Job drawing, mm, ordinate dimensions from the low corner. One solid piece. A direction names the side the tool comes from. Coordinates: 2 decimals unless noted, no trailing zeros. Loops run counter-clockwise (first coordinate to the right, second up) from the corner with the lowest first, then second, coordinate; pieces in that order, holes last. Notation, with made-up numbers: M 61,58 L 117,58 A6 ccw 117,66 Z; hole C -40,47.5 d7. An arc over 180 degrees is marked long. Answer as a JSON object with one key per item and string values. Group by question number.
1. Drill centre lines: L1, parallel to Z at x = 2.5, y = 9; L2, parallel to Z at x = 18.5, y = 13.5; L3, parallel to X at y = 8.95, z = 1.65 (1 decimal). Where is each one in solid material? Low to high.
2. Drop flat-ended pins along their axis: pin 1 Ø8 at (x, z) = (8, 4.5) entering from -Y; pin 2 Ø10 at (x, z) = (23, 3) entering from -Y; pin 3 Ø2 at (x, y) = (7.5, 17) entering from +Z. Give the stop position or say it passes through.
3. 3-axis set-ups, long thin cutter, end or side, ignore diameter. For the marked faces 5, 6 and 7: which of +Z, -Z, +X, -X, +Y, -Y reach the whole face in a straight line?
4. Mould opens along X. For the marked faces 1, 2, 3 and 4 say: released by +X, released by -X, zero draft, split by the parting line, or undercut.
5. Saw through at C-C on y = 20.2. Write the cut outline in (x, z), then the cut area to 3 significant figures.
6. Saw through at A-A on x = 5.25. Write the cut outline in (y, z) (1 decimal).
7. Saw through at D-D on z = 12.75. Write the cut outline in (x, y) (1 decimal).
8. Saw through at B-B on y = 12.7. Write the cut outline in (x, z).
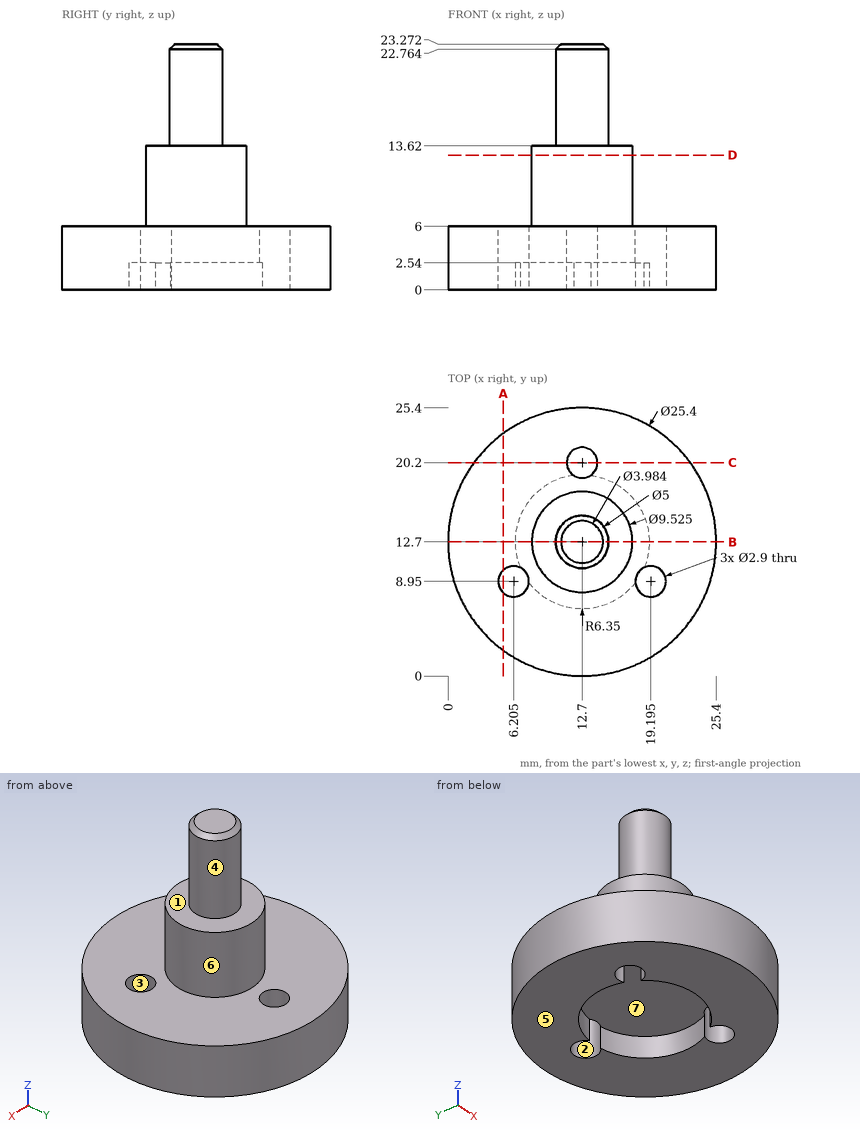
Outcome:
{
 "1": {"L1": "z = 0 to 6", "L2": "z = 2.54 to 6", "L3": "x = 0.6 to 4.8, 20.6 to 24.8"},
 "2": {"pin 1": "stops at y = 0.02", "pin 2": "stops at y = 1.16", "pin 3": "stops at z = 6"},
 "3": {"face 5": "-Z, +X, -X, +Y, -Y", "face 6": "+Z", "face 7": "-Z"},
 "4": {"face 1": "zero draft", "face 2": "undercut", "face 3": "undercut", "face 4": "split by the parting line"},
 "5": {"outline": "M 2.45,0 L 11.25,0 L 11.25,6 L 2.45,6 Z; M 14.15,0 L 22.95,0 L 22.95,6 L 14.15,6 Z", "area": "106 mm²"},
 "6": {"outline": "M 2.4,0 L 7.9,0 L 7.9,6 L 2.4,6 Z; M 10,0 L 23,0 L 23,6 L 10,6 Z"},
 "7": {"outline": "C 12.7,12.7 d9.5"},
 "8": {"outline": "M 0,0 L 6.35,0 L 6.35,2.54 L 19.05,2.54 L 19.05,0 L 25.4,0 L 25.4,6 L 17.46,6 L 17.46,13.62 L 15.2,13.62 L 15.2,22.76 L 14.69,23.27 L 10.71,23.27 L 10.2,22.76 L 10.2,13.62 L 7.94,13.62 L 7.94,6 L 0,6 Z"}
}
